The model under review builds one solid part; all positions refer to its coordinate system, in mm. Face numbers are marked on the shaded views. Coordinates: 2 decimals unless noted, no trailing zeros. Write each loop counter-clockwise with the first axis right and the second up, starting at its lowest first coordinate (ties: lowest second). Pieces come first, ordered by that corner, then holes. Notation, with made-up numbers: M 64,43.25 L 111,43.25 A5 cw 111,51.25 Z; hole C 62.25,79.5 d3. An arc over 180 degrees is marked long. Answer as a JSON object with one key per item and string values.
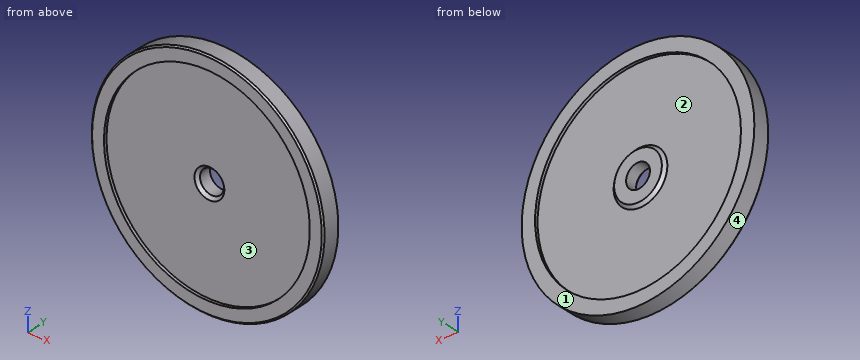
Autodesk Inventor part; units mm, degrees
ref_plane "YZ Plane" through (0, 0, 0) normal (1, 0, 0) x (0, 1, 0)
ref_plane "XZ Plane" through (0, 0, 0) normal (0, 1, 0) x (-1, 0, 0)
ref_plane "XY Plane" through (0, 0, 0) normal (0, 0, 1) x (1, 0, 0)
sketch "Sketch1" plane through (0, 0, 0) normal (0, 0, 1) x (1, 0, 0)
  line L0 (-39, 0) -> (-34.5, 0)
  line L1 (-34.5, 0) -> (-34.5, 1)
  line L2 (-34.5, 1) -> (-4, 1)
  line L3 (-4, 1) -> (-4, 6)
  line L4 (-4, 6) -> (-8, 6)
  line L5 (-8, 6) -> (-8, 5)
  line L6 (-8, 5) -> (-34.5, 5)
  line L7 (-34.5, 5) -> (-34.5, 6)
  line L8 (-34.5, 6) -> (-39, 6)
  line L9 (-39, 6) -> (-39, 0)
  line L10 (0, 0) -> (0, 3.3453)
  line L11 (-34.5, 1) -> (-34.5, 1.25)
  line L12 (-34.5, 1.25) -> (-32.5, 1)
  dimension "d0" = 8
  dimension "d3" = 16
  dimension "d8" = 1
  dimension "d9" = 1
  dimension "d10" = 4
  dimension "d11" = 78
  dimension "d18" = 69
  dimension "d23" = 0.25
  dimension "d24" = 2
revolve "Revolution1" add sketch "Sketch1" angle 360 about axis through (0, 0, 0) along (0, 1, 0)
chamfer "Chamfer1" distance 1 angle 45 2 edges at (4, 1, 0) (8, 5, 0)
chamfer "Chamfer2" distance 0.5 angle 45 1 edges at (39, 0, 0)
properties part number "009" material "Stainless Steel, 440C"
(1) Wall thickness on line 1 along Z through (x, y) = (0, 0.6); line 2 along Z through (x, y) = (0.5, 5.4); line 3 along Z through (x, y) = (0, 3.8): over which ranges is each line inside the solid? List them lowest first. Write a range as from..to.
Results list:
{"line 1": "-39..-34.5, 34.5..39", "line 2": "-39..-34.5, -8.58..-3.97, 3.97..8.58, 34.5..39", "line 3": "-39..-4, 4..39"}
(2) Draft analysis for pull direction X (two halves, no side actions). For the marked faces 1, 2, 3 and 4, state which applies: released by +X, released by -X, zero draft, split by the parting line, or undercut.
Results list:
{"face 1": "zero draft", "face 2": "undercut", "face 3": "undercut", "face 4": "split by the parting line"}
(3) For pin 1 Ø5 at (x, z) = (0, 0) entering from -Y; pin 2 Ø10 at (x, z) = (23.5, 10) entering from +Y; pin 3 Ø6 at (x, z) = (-29.5, -7) entering from -Y; pin 4 Ø3 at (y, z) = (4.5, 16) entering from +X, all flat-tipped, find the tip position at first contact; note any pin that passes through.
Results list:
{"pin 1": "through", "pin 2": "y = 5", "pin 3": "y = 1", "pin 4": "x = 36.2"}
(4) Add section C-C on y = 3.2. Give the boundary of the cut face in (x, z).
Results list:
{"outline": "C 0,0 d78; hole C 0,0 d8"}
